Work out the finished part from the listing and answer in its coordinate system (mm). Give positions to 0.01 mm unless a question says otherwise; leave off trailing zeros. Use one line per item in the form item = value. Start each with the question number.
from build123d import *

# Parameters (mm, degrees)
SKETCH3_R               = 2.032
BOSS_EXTRUDE1_DEPTH     = 914.4
CUT_EXTRUDE1_DEPTH      = 915.510236411
CUT_EXTRUDE1_DEPTH_BACK = 915.510236411
SKETCH4_R               = 0.55245


with BuildPart() as part:
    # Sketch3 → Boss-Extrude1 (new, symmetric)
    with BuildSketch(Plane.XY):
        with BuildLine():
            Line((3.2512, 5.35559), (3.2512, 5.13461))
            ThreePointArc((3.2512, 5.13461), (3.542455946, 4.431455946), (4.24561, 4.1402))
            Line((4.24561, 4.1402), (6.42239, 4.1402))
            ThreePointArc((6.42239, 4.1402), (7.341105046, 3.526334232), (7.125544054, 2.442635946))
            Line((7.125544054, 2.442635946), (3.854875946, -0.828032163))
            ThreePointArc((3.854875946, -0.828032163), (2.887046479, -1.474715138), (1.745413783, -1.7018))
            Line((1.745413783, -1.7018), (0, -1.7018))
            Line((0, -1.7018), (0, -6.35))
            Line((0, -6.35), (10.16, -6.35))
            ThreePointArc((10.16, -6.35), (11.956051224, -5.606051224), (12.7, -3.81))
            Line((12.7, -3.81), (12.7, 3.81))
            ThreePointArc((12.7, 3.81), (11.956051224, 5.606051224), (10.16, 6.35))
            Line((10.16, 6.35), (4.24561, 6.35))
            ThreePointArc((4.24561, 6.35), (3.542455946, 6.058744054), (3.2512, 5.35559))
        make_face()
        with Locations(Location((8.7249, -2.3876, 0), (0, 0, 180))):
            Circle(SKETCH3_R, mode=Mode.SUBTRACT)
    extrude(amount=BOSS_EXTRUDE1_DEPTH, both=True)

    # Sketch4 → Cut-Extrude1 (cut, two sides: drawn at the far end of the back side and taken through both)
    with BuildSketch(Plane.XY.offset(-CUT_EXTRUDE1_DEPTH_BACK)):
        with Locations((5.86994, 6.35)):
            Circle(SKETCH4_R)
        with Locations((10.20445, 6.35)):
            Circle(SKETCH4_R)
        with Locations((5.86994, -6.35)):
            Circle(SKETCH4_R)
        with Locations((10.20445, -6.35)):
            Circle(SKETCH4_R)
    extrude(amount=CUT_EXTRUDE1_DEPTH + CUT_EXTRUDE1_DEPTH_BACK, mode=Mode.SUBTRACT)

    # Mirror1: part across plane


with BuildPart() as part_1:
    add(part.part)
    add(part.part.mirror(Plane(origin=(0, 0, 0), x_dir=(0, 0, 1), z_dir=(1, 0, 0))))


solid = part_1.part
1) Flat-ended cylindrical pins translate along their axes: pin 1 Ø3.5 at (x, y) = (8.72, -2.39) entering from +Z; pin 2 Ø1.7 at (x, z) = (0.5, -422.5) entering from +Y. Find the tip coordinate at first contact, or state that the pin passes through.
2) Find the intervals of material crossed by probe 1 along X at (y, z) = (1.75, -359); probe 2 along Y at (x, z) = (-9, -393.5); probe 3 along X at (y, z) = (1.25, 12), in increasing order.
3) A cutting plane is placed at A-A (z = -196). State how many separate pieces and enclosed holes the cut face has, plus the area to 3 significant figures.
Answer sheet:
q1.pin_1 = through
q1.pin_2 = -1.7
q2.probe_1 = -12.7 to -6.43, 6.43 to 12.7
q2.probe_2 = -6.35 to -4.4, -0.37 to 6.35
q2.probe_3 = -12.7 to -5.93, 5.93 to 12.7
q3.separate_pieces = 1
q3.enclosed_holes = 2
q3.area = 206 mm²
